```python
from build123d import *

# Parameters (mm, degrees)
SKETCH2_W           = 47.5
SKETCH2_H           = 47.5
SKETCH2_R           = 2
SKETCH2_R_2         = 11.5
BOSS_EXTRUDE1_DEPTH = 2
CHAMFER1_SIZE       = 3


with BuildPart() as part:
    # Sketch2 → Boss-Extrude1 (new body)
    with BuildSketch(Plane(origin=(0, 0, 0), x_dir=(1, 0, 0), z_dir=(0, 1, 0))):
        Rectangle(SKETCH2_W, SKETCH2_H)
        with Locations(Location((-15.5, 15.5, 0), (0, 0, 270))):
            Circle(SKETCH2_R, mode=Mode.SUBTRACT)
        with Locations(Location((15.5, 15.5, 0), (0, 0, 270))):
            Circle(SKETCH2_R, mode=Mode.SUBTRACT)
        with Locations(Location((15.5, -15.5, 0), (0, 0, 270))):
            Circle(SKETCH2_R, mode=Mode.SUBTRACT)
        with Locations(Location((-15.5, -15.5, 0), (0, 0, 270))):
            Circle(SKETCH2_R, mode=Mode.SUBTRACT)
        with Locations(Location((0, 0, 0), (0, 0, 270))):
            Circle(SKETCH2_R_2, mode=Mode.SUBTRACT)
    extrude(amount=BOSS_EXTRUDE1_DEPTH)

    # Chamfer1
    chamfer1_edges = [part.edges().sort_by_distance(p)[0] for p in [
        (23.75, 1, 23.75),
        (-23.75, 1, 23.75),
        (-23.75, 1, -23.75),
        (23.75, 1, -23.75),
    ]]
    chamfer(chamfer1_edges, length=CHAMFER1_SIZE)


solid = part.part
```
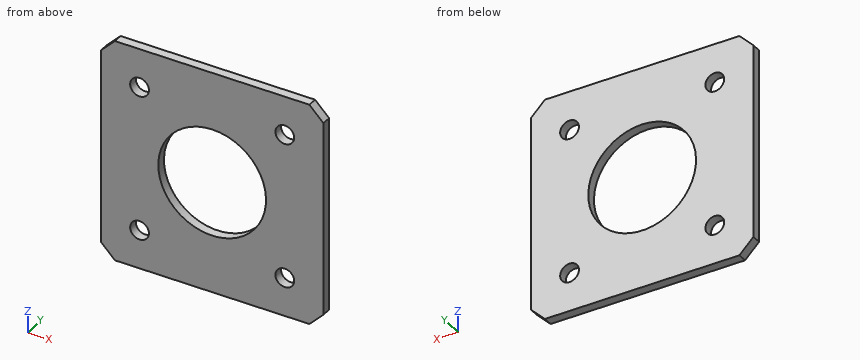
The listing builds one solid part. Answer for the finished solid, in the listing's coordinates (mm). Give positions to 0.01 mm unless a question says otherwise; leave off trailing zeros. Order: outer loops, then holes, each group sorted by start corner. A loop starts at its lowest first (then second) coordinate and runs counter-clockwise, first axis right, second up. Notation, with made-up numbers: (-27.75, 87.5) - (6.25, 87.5) arc R25 ccw to (6.25, 116.5) - close; hole circle Ø6 at (-36.5, 37). An arc over 180 degrees is marked (long way). Use one line per item in the form item = value. Start each with the question number.
(1) A cutting plane is placed at C-C, the plane y = 0.3. Write down the section's boundary in (x, z), then the cut area to 3 significant figures.
(2) A cutting plane is placed at B-B, the plane z = -15.5. Write down the section's boundary in (x, y), then the cut area to 3 significant figures.
(3) Flat-ended cylindrical pins translate along their axes: pin 1 Ø4.5 at (x, z) = (15.5, -15.5) entering from +Y; pin 2 Ø3.5 at (x, z) = (-15.5, 15.5) entering from -Y. Find the tip coordinate at first contact, or state that the pin passes through.
(4) Consider line 1 (X direction, y = 1.55, z = 15.5); line 2 (X direction, y = 0.45, z = 0); line 3 (Z direction, x = -16.5, y = 1.15). Determine where each line is inside the solid, lowest interval first. Write a range as from..to.
(5) A cutting plane is placed at A-A, the plane x = 0. Write down the section's boundary in (y, z).
(6) A cutting plane is placed at D-D, the plane x = 15.5. Write down the section's boundary in (y, z).
Ans:
q1.outline = (-23.75, -20.75) - (-20.75, -23.75) - (20.75, -23.75) - (23.75, -20.75) - (23.75, 20.75) - (20.75, 23.75) - (-20.75, 23.75) - (-23.75, 20.75) - close; hole circle Ø4 at (-15.5, -15.5); hole circle Ø4 at (-15.5, 15.5); hole circle Ø23 at (0, 0); hole circle Ø4 at (15.5, -15.5); hole circle Ø4 at (15.5, 15.5)
q1.area = 1,770 mm^2
q2.outline = (-23.75, 0) - (-17.5, 0) - (-17.5, 2) - (-23.75, 2) - close; (-13.5, 0) - (13.5, 0) - (13.5, 2) - (-13.5, 2) - close; (17.5, 0) - (23.75, 0) - (23.75, 2) - (17.5, 2) - close
q2.area = 79.0 mm^2
q3.pin_1 = 2
q3.pin_2 = through
q4.line_1 = -23.75..-17.5, -13.5..13.5, 17.5..23.75
q4.line_2 = -23.75..-11.5, 11.5..23.75
q4.line_3 = -23.75..-17.23, -13.77..13.77, 17.23..23.75
q5.outline = (0, -23.75) - (2, -23.75) - (2, -11.5) - (0, -11.5) - close; (0, 11.5) - (2, 11.5) - (2, 23.75) - (0, 23.75) - close
q6.outline = (0, -23.75) - (2, -23.75) - (2, -17.5) - (0, -17.5) - close; (0, -13.5) - (2, -13.5) - (2, 13.5) - (0, 13.5) - close; (0, 17.5) - (2, 17.5) - (2, 23.75) - (0, 23.75) - close
